Read the model definition and answer for the solid it produces. Units are mm, in the model's axes. A direction names the side the tool comes from. Round coordinates to 2 decimals unless told otherwise and drop trailing zeros. Order: outer loops, then holes, each group sorted by start corner. A loop starts at its lowest first (then second) coordinate and runs counter-clockwise, first axis right, second up.
from build123d import *

# Parameters (mm, degrees)
F0_W     = 76.2
F0_H     = 129.54
F1_DEPTH = 46.99
F2_R     = 37.2745
F3_DEPTH = 129.54
F4_W     = 3.175
F4_H     = 7.62
F4_W_2   = 2.777509
F5_DEPTH = 76.2


with BuildPart() as f1:
    # F0 (on Front) → F1 (new body)
    with BuildSketch(Plane.XZ):
        with Locations((0, 64.77)):
            Rectangle(F0_W, F0_H)
    extrude(amount=F1_DEPTH)

    # F2 (on Top) → F3 (cut, through all)
    with BuildSketch(Plane.XY):
        Circle(F2_R)
    extrude(amount=F3_DEPTH, mode=Mode.SUBTRACT)

    # F4 (on face) → F5 (cut, through all)
    with BuildSketch(Plane(origin=(-38.1, 0, 0), x_dir=(0, -1, 0), z_dir=(-1, 0, 0))):
        with Locations((42.8625, 29.21)):
            Rectangle(F4_W, F4_H)
        with Locations((42.663754, 100.33)):
            Rectangle(F4_W_2, F4_H)
    extrude(amount=-F5_DEPTH, mode=Mode.SUBTRACT)


solid = f1.part
Q1. For faces 1 (the face through (-1, -46.99, 66)), 2 (the face through (-1, -43, 96.52)), determine the directions among +Z, -Z, +X, -X, +Y, -Y from which every point of the face is accessible in a straight line to the end or side of a thin tool.
Outcome:
face 1: +Z, -Z, +X, -X, -Y
face 2: +X, -X
Q2. Flat-ended cylindrical pins translate along their axes: pin 1 (10 mm diameter, centred on x = -22, z = 33.5, fed in from +Y); pin 2 (1.4 mm diameter, centred on x = -14.5, y = -43.5, fed in from -Z); pin 3 (2.5 mm diameter, centred on x = -9, z = 29, fed in from +Y); pin 4 (4 mm diameter, centred on x = 13, z = 101.5, fed in from +Y). Find the tip coordinate at first contact, or state that the pin passes through.
Outcome:
pin 1: stops at y = -25.7
pin 2: stops at z = 0
pin 3: stops at y = -35.84
pin 4: stops at y = -34.12
Q3. A cutting plane is placed at D-D, the plane z = 8. Give the vertices of the cut face in (x, y).
Outcome:
outline: (-38.1, -46.99) - (38.1, -46.99) - (38.1, 0) - (37.27, 0) arc R37.27 cw to (-37.27, 0) - (-38.1, 0) - close
Q4. Straight lines are drawn through the part: probe 1 along Z at (x, y) = (-24, -42); probe 2 along X at (y, z) = (-23.5, 70); probe 3 along X at (y, z) = (-16.5, 116). For each, find the intervals that lie inside material, in ascending order.
Outcome:
probe 1: z = 0 to 25.4, 33.02 to 96.52, 104.14 to 129.54
probe 2: x = -38.1 to -28.93, 28.93 to 38.1
probe 3: x = -38.1 to -33.42, 33.42 to 38.1
Q5. For a pull along Y with two mould halves and no side action, classify faces 3 (the face through (-0.82, -37.265, 63.863)), 4 (the face through (-1, -43, 104.14)), 5 (the face through (-38.1, -23, 64)) as released by +Y, released by -Y, zero draft, split by the parting line, or undercut.
Outcome:
face 3: released by +Y
face 4: undercut
face 5: zero draft
Q6. A cutting plane is placed at B-B, the plane x = 0. Give the number of separate pieces and of enclosed holes in the cut face, plus the area to 3 significant figures.
Outcome:
separate pieces: 1
enclosed holes: 2
area: 1,210 mm2
Q7. A cutting plane is placed at C-C, the plane y = -36. Give the vertices of the cut face in (x, z).
Outcome:
outline: (-38.1, 0) - (-9.66, 0) - (-9.66, 129.54) - (-38.1, 129.54) - close; (9.66, 0) - (38.1, 0) - (38.1, 129.54) - (9.66, 129.54) - close
